Read the model definition and answer for the solid it produces. Units are mm, in the model's axes. Give positions to 0.01 mm unless a question says otherwise; leave off trailing zeros. Order: outer loops, then holes, each group sorted by start corner. A loop starts at its lowest first (then second) coordinate and runs counter-clockwise, first axis right, second up. Notation, with made-up numbers: (-32.75, -8.5) - (6.25, -8.5) arc R15 cw to (6.25, -0.5) - close; hole circle Ø1 at (36, 85.25). An arc over 180 degrees is marked (long way). Use a Markdown table: item, result. Add a question column.
1. Consider L1, parallel to X at y = -21, z = 1.1; L2, parallel to X at y = 24, z = 0.1; L3, parallel to X at y = 7.5, z = 1.35. Determine where each line is inside the solid, lowest interval first.
2. A cutting plane is placed at B-B on x = -84.5. Determine the outline of the cut face in (y, z), and give its area (3 significant figures).
3. A cutting plane is placed at C-C on x = -125.5. Determine the outline of the cut face in (y, z).
4. A flat-ended cylindrical pin translates along its axis: P1, Ø3.5, axis at x = 88.99, y = 9.5, coming from the -Z side. Find the tip coordinate at first contact, or state that the pin passes through.
5. A cutting plane is placed at A-A on z = 0.7. State how many separate pieces and enclosed holes the cut face has, and give its area (3 significant figures).
Autodesk Inventor part; units mm, degrees
ref_plane "YZ Plane" through (0, 0, 0) normal (1, 0, 0) x (0, 1, 0)
ref_plane "XZ Plane" through (0, 0, 0) normal (0, 1, 0) x (-1, 0, 0)
ref_plane "XY Plane" through (0, 0, 0) normal (0, 0, 1) x (1, 0, 0)
sketch "Sketch1" plane through (0, 0, 0) normal (0, 0, 1) x (1, 0, 0)
  circle A0 centre (-133.2579, -22.248) radius 2.1844
  circle A1 centre (-101.5079, -0.023) radius 2.2225
  circle A2 centre (-44.3579, -22.248) radius 2.1844
  circle A3 centre (25.4921, 9.502) radius 2.1844
  circle A4 centre (25.4921, 22.202) radius 2.1844
  circle A5 centre (88.9921, 9.502) radius 2.1844
  circle A6 centre (88.9921, 22.202) radius 2.1844
  circle A7 centre (44.5421, -22.248) radius 2.1844
  circle A8 centre (133.4421, -22.248) radius 2.1844
  line L0 (133.4421, -22.248) -> (171.5421, -22.248)
  line L1 (171.5421, -22.248) -> (171.5421, -60.348)
  line L2 (171.5421, -60.348) -> (-184.0579, -60.348)
  line L3 (-184.0579, -60.348) -> (-184.0579, -9.548)
  line L4 (-184.0579, -9.548) -> (-114.2079, -9.548)
  line L5 (-114.2079, -9.548) -> (-114.2079, 6.327)
  line L6 (-19.3781, 6.327) -> (-19.3781, 31.727)
  line L7 (-19.3781, 31.727) -> (6.4421, 31.727)
  line L8 (-19.3781, 6.327) -> (6.4421, 31.727)
  line L9 (6.4421, 31.727) -> (108.0421, 31.727)
  line L10 (108.0421, 31.727) -> (133.1583, 6.1953)
  line L11 (171.5421, -22.248) -> (108.0421, 31.727)
  line L12 (88.9921, 22.202) -> (108.0421, 22.202)
  line L13 (108.0421, 22.202) -> (108.0421, 31.727)
  line L14 (25.4921, 22.202) -> (6.4421, 22.202)
  line L15 (6.4421, 22.202) -> (6.4421, 31.727)
  line L16 (-19.3781, 6.327) -> (-101.5079, 6.327)
  line L17 (-101.5079, 6.327) -> (-114.2079, -9.548)
  line L18 (171.5421, -22.248) -> (171.5421, -9.548)
  line L19 (171.5421, -9.548) -> (108.0421, 31.727)
  line L20 (-114.2079, -9.548) -> (-120.5579, -9.548)
  line L21 (-101.5079, 6.327) -> (-107.8579, 6.327)
  line L22 (-107.8579, 6.327) -> (-120.5579, -9.548)
  line L23 (171.5421, -60.348) -> (171.5421, -64.6152)
  line L24 (171.5421, -64.6152) -> (-184.0579, -64.6152)
  line L25 (-184.0579, -64.6152) -> (-184.0579, -60.348)
  point P0 (0, 0)
  dimension "d0" = 38.1
  dimension "d1" = 38.1
  dimension "d2" = 355.6
  dimension "d3" = 50.8
  dimension "d4" = 69.85
  dimension "d5" = 15.875
  dimension "d7" = 25.4
  dimension "d10" = 19.05
  dimension "d11" = 19.05
  dimension "d14" = 12.7
  dimension "d17" = 6.35
  dimension "d18" = 6.35
  dimension "d21" = 4.2672
extrude "Extrusion2" add sketch "Sketch1" along normal blind 1.5875 contours L1 L2 L3 L4 L17 L16 L8 L9 L11 | L23 L24 L25 L2 | L22 L5 L4 | L17 L5 L22 L21
extrude "Extrusion3" add sketch "Sketch1" along normal blind 1.5875 contours L11 L19 L18
fillet "Fillet1" radius 8.4667 3 edges at (-107.8579, 6.327, 0.7937) (6.4421, 31.727, 0.7937) (-19.3781, 6.327, 0.7937)
fillet "Fillet2" radius 8.4667 3 edges at (108.0421, 31.727, 0.7937) (171.5421, -9.548, 0.7937) (-184.0579, -9.548, 0.7937)
fillet "Fillet3" radius 6.35 2 edges at (171.5421, -64.6152, 0.7937) (-184.0579, -64.6152, 0.7937)
properties part number "Skirt"
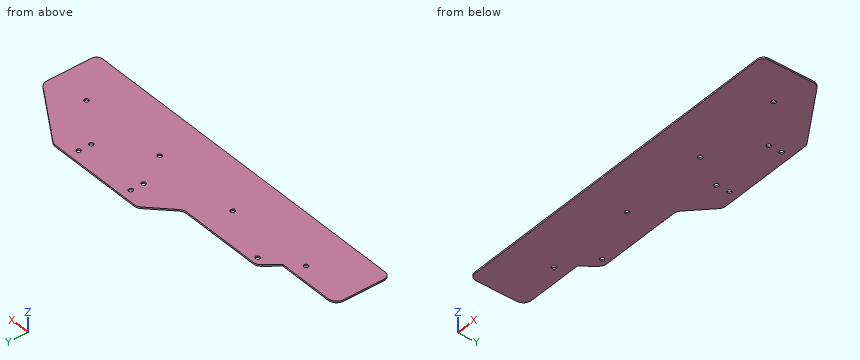
Output values:
| question | item | result |
|---|---|---|
| 1 | L1 | -184.06 to -135.05, -131.47 to -46.15, -42.57 to 42.75, 46.33 to 131.65, 135.23 to 171.54 |
| 1 | L2 | -1.41 to 24.25, 26.73 to 87.75, 90.23 to 119.93 |
| 1 | L3 | -18.54 to 24.62, 26.37 to 88.12, 89.87 to 145.31 |
| 2 | outline | (-64.62, 0) - (6.33, 0) - (6.33, 1.59) - (-64.62, 1.59) - close |
| 2 | area | 113 mm² |
| 3 | outline | (-64.62, 0) - (-9.55, 0) - (-9.55, 1.59) - (-64.62, 1.59) - close |
| 4 | P1 | through |
| 5 | separate pieces | 1 |
| 5 | enclosed holes | 9 |
| 5 | area | 27,200 mm² |
